Geometry check sheet. Reference: drawing and pictorial views, mm from the part's lowest x, y, z. A direction names the side the tool comes from. Round coordinates to 2 decimals unless told otherwise and drop trailing zeros. Order: outer loops, then holes, each group sorted by start corner. A loop starts at its lowest first (then second) coordinate and runs counter-clockwise, first axis right, second up.
(1) Sectioned sample at A-A, the plane x = 10.5. Enter the section's corners in (y, z) (3 decimals), and give its area (3 significant figures).
(2) Tool access check on the marked faces 1 and 2. Record the directions out of +Z, -Z, +X, -X, +Y, -Y that give a thin tool (end or side, any length) a straight path to the whole face; none if there is none.
(3) Sectioned sample at B-B, the plane y = 30. Enter the section's corners in (x, z).
(4) Sectioned sample at C-C, the plane x = 36.5. Enter the section's corners in (y, z).
(5) Thickness scan on probe 1 along Z at (x, y) = (6, 22.5). Record the ranges inside material, lowest first.
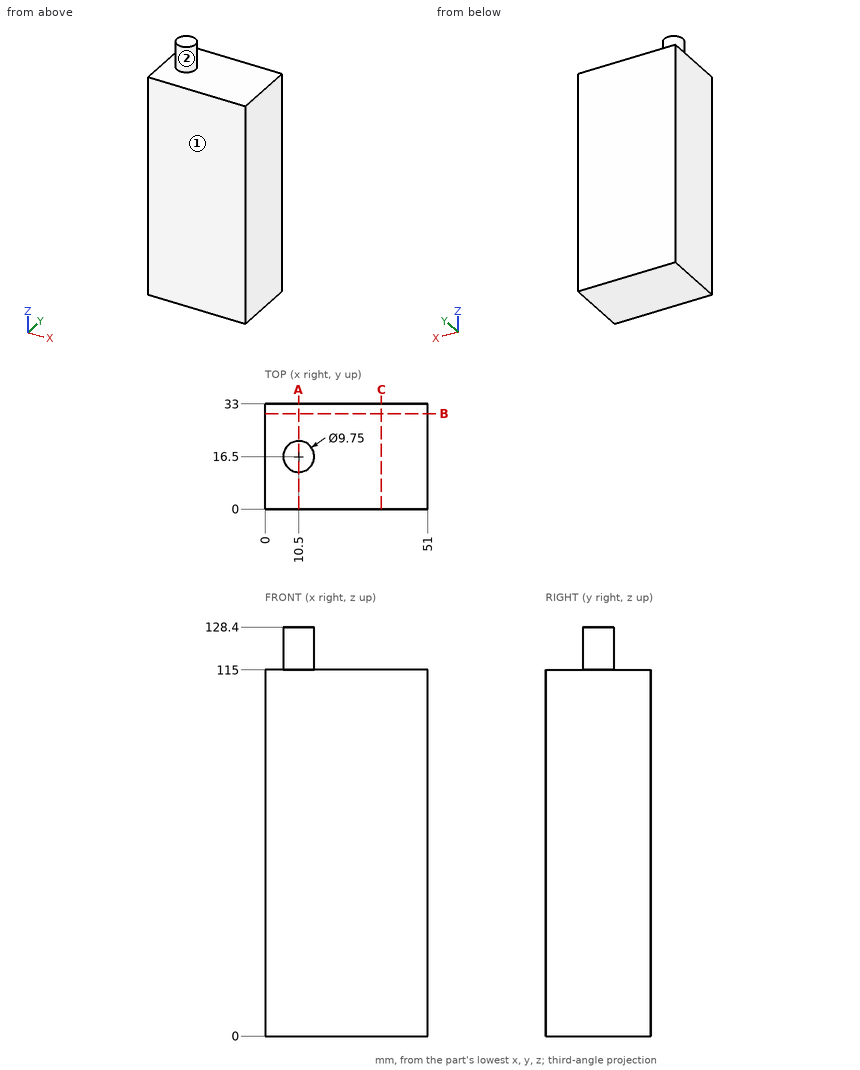
Derived:
1. outline: (0, 0) - (33, 0) - (33, 115) - (21.375, 115) - (21.375, 128.4) - (11.625, 128.4) - (11.625, 115) - (0, 115) - close
1. area: 3,930 mm2
2. face 1: +Z, -Z, +X, -X, -Y
2. face 2: +Z
3. outline: (0, 0) - (51, 0) - (51, 115) - (0, 115) - close
4. outline: (0, 0) - (33, 0) - (33, 115) - (0, 115) - close
5. probe 1: z = 0 to 115
